Input: dimensioned drawing with shaded views. Units: mm. Origin: part minimum x, y, z. A direction names the side the tool comes from. Round coordinates to 2 decimals unless told otherwise and drop trailing zeros. Loops run counter-clockwise (first coordinate to the right, second up) from the corner with the lowest first, then second, coordinate; pieces in that order, holes last. Notation, with made-up numbers: M 53.25,-39 L 107.25,-39 A26 ccw 107.25,0 Z; hole C -20,17 d11. An arc over 180 degrees is marked long. Put each result on its own line as item: value. Start each with the question number.
1) Reachability of the marked faces 1, 2, 3 and 4 from +Z, -Z, +X, -X, +Y, -Y: full face, straight path, thin tool, end or side. Return the list, or none.
2) Line query: probe 1 along Y at (x, z) = (57.15, 59.5) (1 decimal); probe 2 along Z at (x, y) = (65.5, 25.5) (1 decimal); probe 3 along X at (y, z) = (38, 57) (1 decimal). Output: solid intervals per line, ascending.
3) Draft query along Z for the marked faces 5, 6 and 7. Return one class per face: +Z half, -Z half, draft (parallel to the pull), parting line (faces both ways), or undercut.
4) Section C-C on x = 44. Output: boundary loops of the cut face in (y, z) (1 decimal).
5) Section A-A on y = 12.7. State how many separate pieces and enclosed holes the cut face has, plus the area to 3 significant figures.
6) Pin query (flat end, axial travel): pin 1 (11 mm diameter, centred on x = 15.88, z = 61.91, fed in from -Y); pin 2 (7.5 mm diameter, centred on x = 57.15, y = 63.5, fed in from +Z); pin 3 (2 mm diameter, centred on y = 38, z = 70, fed in from -X); pin 4 (15 mm diameter, centred on y = 63.5, z = 37, fed in from -X). Return the tip coordinate at first contact, or that it passes through.
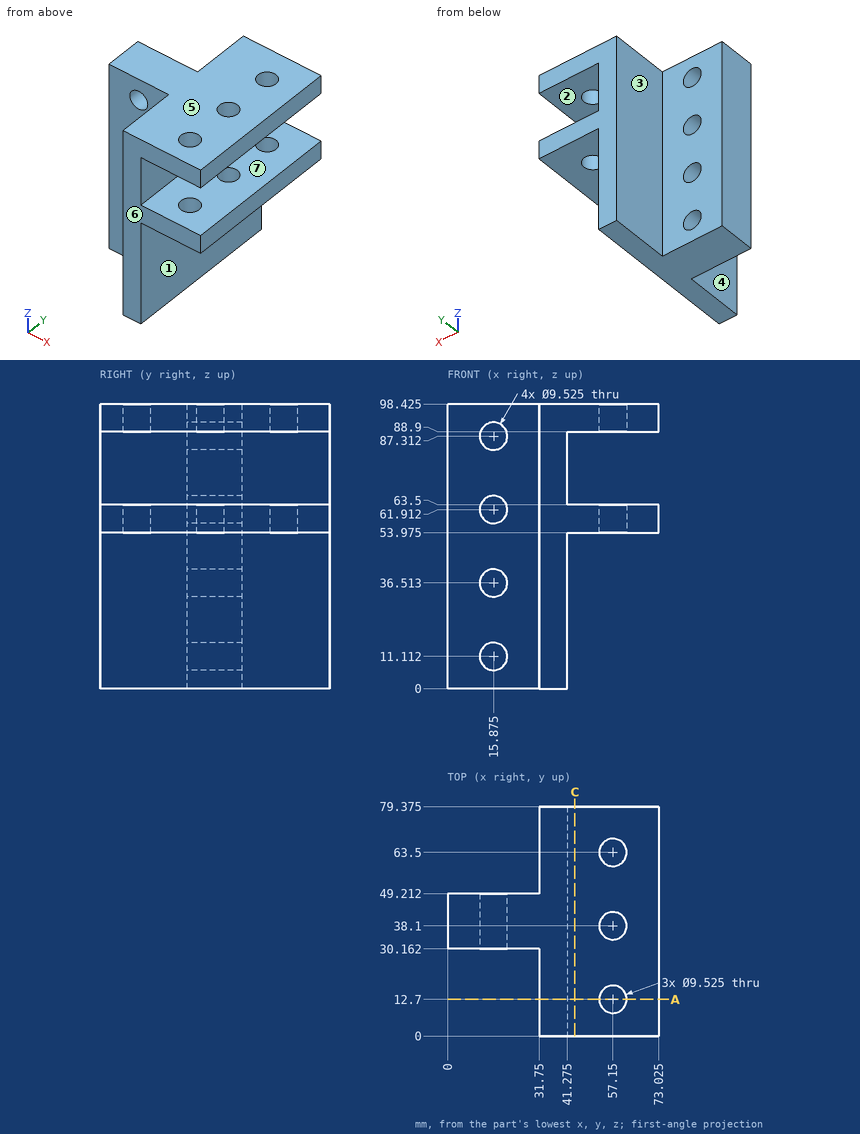
Geometry results:
1. face 1: -Z, +X, +Y, -Y
1. face 2: +X, +Y, -Y
1. face 3: +Z, -Z, -X, +Y
1. face 4: +Z, -Z, -X, -Y
2. probe 1: y = 0 to 7.9, 17.5 to 33.3, 42.9 to 58.7, 68.3 to 79.4
2. probe 2: z = 54 to 63.5, 88.9 to 98.4
2. probe 3: x = 0 to 52.4, 61.9 to 73
3. face 5: +Z half
3. face 6: draft
3. face 7: undercut
4. outline: M 0,54 L 79.4,54 L 79.4,63.5 L 0,63.5 Z; M 0,88.9 L 79.4,88.9 L 79.4,98.4 L 0,98.4 Z
5. separate pieces: 3
5. enclosed holes: 0
5. area: 1,360 mm²
6. pin 1: stops at y = 30.16
6. pin 2: passes through
6. pin 3: stops at x = 0
6. pin 4: stops at x = 31.75
